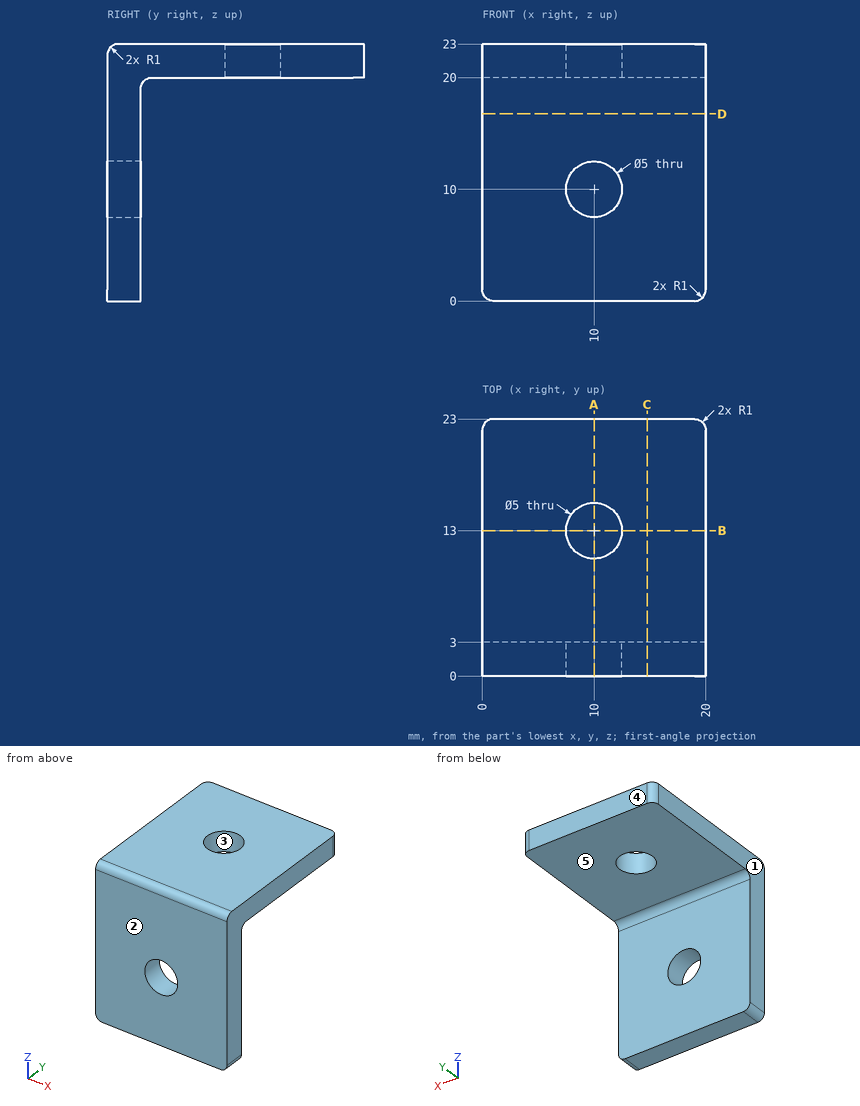
Design review of the part shown in the three views and the two pictorial views. Dimensions are in mm from the part's minimum x, y and z. A direction names the side the tool comes from. Give positions to 0.01 mm unless a question says otherwise; leave off trailing zeros. Loops run counter-clockwise (first coordinate to the right, second up) from the corner with the lowest first, then second, coordinate; pieces in that order, holes last. Notation, with made-up numbers: (43, -33.5) - (60, -33.5) arc R23 ccw to (60, 2.5) - close; hole circle Ø5 at (54, 89.25). An arc over 180 degrees is marked (long way). Answer as a JSON object with one key per item and string values.
Q1. Add section C-C on x = 14.75. State the section outline as (y, z) points.
Worked out:
{"outline": "(0, 0) - (3, 0) - (3, 19) arc R1 cw to (4, 20) - (23, 20) - (23, 23) - (1, 23) arc R1 ccw to (0, 22) - close"}
Q2. To check wall thickness, follow line 1 along X through (y, z) = (1.1, 10); line 2 along Y through (x, z) = (6.5, 18); line 3 along Z through (x, y) = (5.5, 20.5). State the ranges of each line that lie inside material, in increasing order.
Worked out:
{"line 1": "x = 0 to 7.5, 12.5 to 20", "line 2": "y = 0 to 3", "line 3": "z = 20 to 23"}
Q3. Add section B-B on y = 13. State the section outline as (x, z) points, plus the area to 3 significant figures.
Worked out:
{"outline": "(0, 20) - (7.5, 20) - (7.5, 23) - (0, 23) - close; (12.5, 20) - (20, 20) - (20, 23) - (12.5, 23) - close", "area": "45.0 mm^2"}
Q4. Insertion check: pin 1 (4 mm diameter, centred on x = 10, y = 13, fed in from -Z); pin 2 (5.5 mm diameter, centred on x = 13, z = 12.5, fed in from +Y); pin 3 (9.5 mm diameter, centred on x = 5, y = 13, fed in from -Z). Each pin has a flat end and moves straight along its axis. Give the tip position at first contact, or say it passes through.
Worked out:
{"pin 1": "passes through", "pin 2": "stops at y = 3", "pin 3": "stops at z = 20"}
Q5. Mouldability with a two-part tool opening along X and no side actions: class the marked faces 1, 2 and 3 as +X half, -X half, draft (parallel to the pull), parting line (faces both ways), or undercut.
Worked out:
{"face 1": "-X half", "face 2": "draft", "face 3": "undercut"}
Q6. For the marked faces 4 and 5, list the 3-axis set-ups (+Z, -Z, +X, -X, +Y, -Y) from which the entire face can be reached by the end or side of a thin tool; tool diameter is ignored.
Worked out:
{"face 4": "+Z, -Z, +X, -X, +Y", "face 5": "-Z, +X, -X, +Y"}
Q7. Add section A-A on x = 10. State the section outline as (y, z) points.
Worked out:
{"outline": "(0, 0) - (3, 0) - (3, 7.5) - (0, 7.5) - close; (0, 12.5) - (3, 12.5) - (3, 19) arc R1 cw to (4, 20) - (10.5, 20) - (10.5, 23) - (1, 23) arc R1 ccw to (0, 22) - close; (15.5, 20) - (23, 20) - (23, 23) - (15.5, 23) - close"}
Q8. Add section D-D on z = 16.75. State the section outline as (x, y) points.
Worked out:
{"outline": "(0, 0) - (20, 0) - (20, 3) - (0, 3) - close"}
